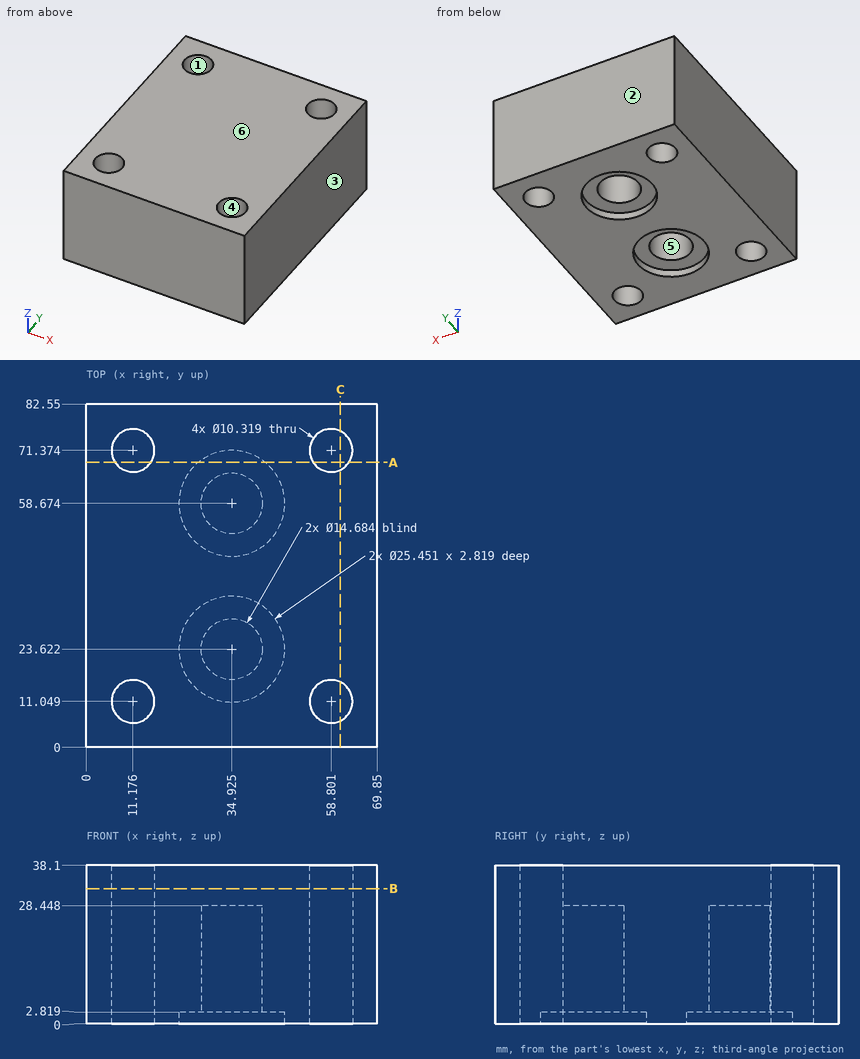
Answer from the drawing. Dimensions are ordinates in mm from the lowest x, y and z of the part. A direction names the side the tool comes from. Round coordinates to 2 decimals unless told otherwise and drop trailing zeros. Write each loop counter-clockwise with the first axis right and the second up, starting at its lowest first coordinate (ties: lowest second). Pieces come first, ordered by that corner, then holes. Notation, with made-up numbers: M -25,29.5 L 16,29.5 A31 cw 16,58.5 Z; hole C 29.25,-36 d9. An arc over 180 degrees is marked long. One line per item, written item: value.
Q1. Find section C-C on x = 61. Write down the section's boundary in (y, z).
Data:
outline: M 0,0 L 6.38,0 L 6.38,38.1 L 0,38.1 Z; M 15.72,0 L 66.71,0 L 66.71,38.1 L 15.72,38.1 Z; M 76.04,0 L 82.55,0 L 82.55,38.1 L 76.04,38.1 Z
Q2. Which of the six approach directions +Z, -Z, +X, -X, +Y, -Y give full straight-line access (tool end or side, diameter ignored) to the marked faces 5 and 6?
Data:
face 5: -Z
face 6: +Z, +X, -X, +Y, -Y
Q3. Flat-ended cylindrical pins translate along their axes: pin 1 Ø20.5 at (x, y) = (34.925, 58.674) entering from -Z; pin 2 Ø4.5 at (x, y) = (32.5, 62) entering from -Z; pin 3 Ø6 at (x, y) = (58.801, 71.374) entering from -Z. Find the tip coordinate at first contact, or state that the pin passes through.
Data:
pin 1: z = 2.82
pin 2: z = 28.45
pin 3: through
Q4. For a pull along X with two mould halves and no side action, classify the marked faces 1, 2, 3 and 4 as +X half, -X half, draft (parallel to the pull), parting line (faces both ways), or undercut.
Data:
face 1: undercut
face 2: draft
face 3: +X half
face 4: undercut
Q5. Straight lines are drawn through the part: line 1 (Y direction, x = 31, z = 3); line 2 (Z direction, x = 37.5, y = 20.5); line 3 (X direction, y = 63.5, z = 10.5). For each, find the intervals that lie inside material, in ascending order. Write a range as [from, to].
Data:
line 1: [0, 17.42], [29.83, 52.47], [64.88, 82.55]
line 2: [28.45, 38.1]
line 3: [0, 29.39], [40.46, 69.85]
Q6. Find section A-A on y = 68.5. Count the separate pieces of the cut face and the enclosed holes in it, plus the area to 3 significant figures.
Data:
separate pieces: 3
enclosed holes: 0
area: 1,960 mm2
Q7. Find section B-B on z = 32.5. Write down the section's boundary in (x, y).
Data:
outline: M 0,0 L 69.85,0 L 69.85,82.55 L 0,82.55 Z; hole C 11.18,11.05 d10.32; hole C 11.18,71.37 d10.32; hole C 58.8,11.05 d10.32; hole C 58.8,71.37 d10.32
